Geometry: final body of the model. Coordinates: model frame, mm. A direction names the side the tool comes from. Give positions to 0.01 mm unless a question says otherwise; leave off trailing zeros. Write each loop counter-clockwise with the first axis right and the second up, starting at its lowest first coordinate (ties: lowest second). Pieces come first, ordered by that corner, then holes.
```python
from build123d import *

# Parameters (mm, degrees)
SKETCH1_R           = 57
BOSS_EXTRUDE1_DEPTH = 4
BOSS_EXTRUDE2_START = 8
BOSS_EXTRUDE2_DEPTH = 8
M6_TAPPED_HOLE1_D   = 5


# Read off the part's stored shape, not the designer's step: M4 Tapped Hole1
with BuildPart() as part:
    # Sketch1 → Boss-Extrude1 (new, symmetric)
    with BuildSketch(Plane(origin=(0, 0, 0), x_dir=(1, 0, 0), z_dir=(0, 1, 0))):
        with Locations(Location((0, 0, 0), (0, 0, 270))):
            Circle(SKETCH1_R)
    extrude(amount=BOSS_EXTRUDE1_DEPTH, both=True)

    # Sketch2 → Boss-Extrude2 (add)
    with BuildSketch(Plane(origin=(0, 4, 0), x_dir=(1, 0, 0), z_dir=(0, 1, 0)).offset(BOSS_EXTRUDE2_START)):
        with BuildLine():
            Line((-22.5, -52.37127075), (-22.5, 52.37127075))
            ThreePointArc((-22.5, 52.37127075), (-23.756914523, 51.81321272), (-25, 51.224993899))
            Line((-25, 51.224993899), (-25, -51.224993899))
            ThreePointArc((-25, -51.224993899), (-23.756914523, -51.81321272), (-22.5, -52.37127075))
        make_face()
        with BuildLine():
            ThreePointArc((-15, 54.990908339), (-16.254254993, 54.633315794), (-17.5, 54.247119739))
            Line((-17.5, 54.247119739), (-17.5, -54.247119739))
            ThreePointArc((-17.5, -54.247119739), (-16.254254993, -54.633315794), (-15, -54.990908339))
            Line((-15, -54.990908339), (-15, 54.990908339))
        make_face()
        with BuildLine():
            Line((25, -51.224993899), (25, 51.224993899))
            ThreePointArc((25, 51.224993899), (23.756914523, 51.81321272), (22.5, 52.37127075))
            Line((22.5, 52.37127075), (22.5, -52.37127075))
            ThreePointArc((22.5, -52.37127075), (23.756914523, -51.81321272), (25, -51.224993899))
        make_face()
        with BuildLine():
            ThreePointArc((17.5, 54.247119739), (16.254254993, 54.633315794), (15, 54.990908339))
            Line((15, 54.990908339), (15, -54.990908339))
            ThreePointArc((15, -54.990908339), (16.254254993, -54.633315794), (17.5, -54.247119739))
            Line((17.5, -54.247119739), (17.5, 54.247119739))
        make_face()
    extrude(amount=-BOSS_EXTRUDE2_DEPTH)

    # M6 Tapped Hole1 (through all)
    with Locations(Plane(origin=(0, -4, 0), x_dir=(-1, 0, 0), z_dir=(0, -1, 0))):
        with Locations((0, 0)):
            Hole(M6_TAPPED_HOLE1_D / 2)

    # M4 Tapped Hole1 outline → M4 Tapped Hole1 (revolve, cut)
    with BuildSketch(Plane.XZ):
        Polygon((1.65, -57.000012834), (1.65, -46.9), (0, -45.908579979), (0, -57.000012834), align=None)
        Polygon((0, 57.000003302), (0, 45.908579979), (1.65, 46.9), (1.65, 57.000003302), align=None)
    revolve(axis=Axis((0, 0, 0), (0, 0, 1)), mode=Mode.SUBTRACT)

    # M4 Tapped Hole1 2 outline → M4 Tapped Hole1 2 (revolve, cut)
    with BuildSketch(Plane.YX):
        Polygon((0, 45.908579979), (1.65, 46.9), (1.65, 57.000003302), (0, 57.000003302), align=None)
        Polygon((1.65, -46.9), (0, -45.908579979), (0, -57.000003302), (1.65, -57.000003302), align=None)
    revolve(axis=Axis((0, 0, 0), (1, 0, 0)), mode=Mode.SUBTRACT)


solid = part.part
```
Item 1: Section B-B, the plane z = 49. Return the cut outline in (x, y).
Found:
outline: (-29.12, -4) - (29.12, -4) - (29.12, 4) - (25, 4) - (25, 12) - (22.5, 12) - (22.5, 4) - (17.5, 4) - (17.5, 12) - (15, 12) - (15, 4) - (-15, 4) - (-15, 12) - (-17.5, 12) - (-17.5, 4) - (-22.5, 4) - (-22.5, 12) - (-25, 12) - (-25, 4) - (-29.12, 4) - close; hole circle Ø3.3 at (0, 0)
Item 2: Reachability of faces 1 (the face through (-12, -4, -1)), 2 (the face through (-25, 8, -1)), 3 (the face through (38, 4, -1)), 4 (the face through (-1.216, 1.115, 52.021)), 5 (the face through (-20, 4, -1)) from +Z, -Z, +X, -X, +Y, -Y: full face, straight path, thin tool, end or side. Return the list, or none.
Found:
face 1: +Z, -Z, +X, -X, -Y
face 2: +Z, -Z, -X, +Y
face 3: +Z, -Z, +X, +Y
face 4: +Z
face 5: +Z, -Z, +Y
Item 3: Section A-A, the plane z = -25. Return the cut outline in (x, y) (3 decimals).
Found:
outline: (-51.225, -4) - (51.225, -4) - (51.225, 4) - (25, 4) - (25, 12) - (22.5, 12) - (22.5, 4) - (17.5, 4) - (17.5, 12) - (15, 12) - (15, 4) - (-15, 4) - (-15, 12) - (-17.5, 12) - (-17.5, 4) - (-22.5, 4) - (-22.5, 12) - (-25, 12) - (-25, 4) - (-51.225, 4) - close
Item 4: Section C-C, the plane x = 20. Return the cut outline in (y, z).
Found:
outline: (-4, -53.38) - (4, -53.38) - (4, 53.38) - (-4, 53.38) - close
Item 5: Pull-direction query (Z, two-part tool) for faces 6 (the face through (-46.067, -0.034, 0.261)), 7 (the face through (-0.034, 0.261, -46.067)), 8 (the face through (24, 12, -1)); classes: +Z half, -Z half, draft (parallel to the pull), parting line (faces both ways), or undercut.
Found:
face 6: undercut
face 7: -Z half
face 8: draft
Item 6: Pin query (flat end, axial travel): pin 1 Ø2 at (y, z) = (0, 0) entering from +X; pin 2 Ø9 at (y, z) = (6.5, -12) entering from -X; pin 3 Ø5.5 at (y, z) = (0, 0) entering from +X; pin 4 Ø8 at (x, z) = (-8, -2) entering from +Y. Return the tip coordinate at first contact, or that it passes through.
Found:
pin 1: stops at x = 46.51
pin 2: stops at x = -56.4
pin 3: stops at x = 57
pin 4: stops at y = 4
Item 7: Line query: L1, parallel to X at y = 9.75, z = -10; L2, parallel to Y at x = 54, z = 0; L3, parallel to Z at x = 53, y = 0. Output: solid intervals per line, ascending.
Found:
L1: x = -25 to -22.5, -17.5 to -15, 15 to 17.5, 22.5 to 25
L2: y = -4 to -1.65, 1.65 to 4
L3: z = -20.98 to -1.65, 1.65 to 20.98
Item 8: Section D-D, the plane z = -43. Return the cut outline in (x, y), plus the area to 3 significant figures.
Found:
outline: (-37.42, -4) - (37.42, -4) - (37.42, 4) - (25, 4) - (25, 12) - (22.5, 12) - (22.5, 4) - (17.5, 4) - (17.5, 12) - (15, 12) - (15, 4) - (-15, 4) - (-15, 12) - (-17.5, 12) - (-17.5, 4) - (-22.5, 4) - (-22.5, 12) - (-25, 12) - (-25, 4) - (-37.42, 4) - close
area: 679 mm2
